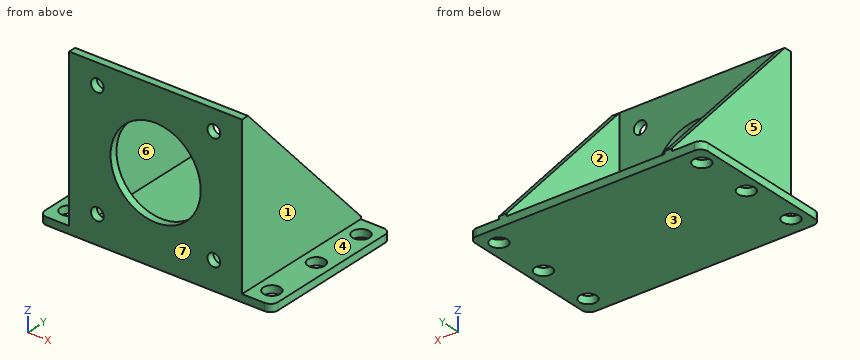
from build123d import *

# Parameters (mm, degrees)
F0_R     = 2.25
F1_DEPTH = 2
F2_W     = 46
F2_H     = 44
F2_R     = 1.7
F2_R_2   = 12
F3_DEPTH = 2
F5_DEPTH = 2
F6_START = -44
F6_DEPTH = 2


with BuildPart() as f1:
    # F0 (on Top) → F1 (new body)
    with BuildSketch(Plane.XY):
        with BuildLine():
            ThreePointArc((0, 2), (0.5857864376, 0.5857864376), (2, 0))
            Line((2, 0), (60, 0))
            ThreePointArc((60, 0), (61.4142135624, 0.5857864376), (62, 2))
            Line((62, 2), (62, 38))
            ThreePointArc((62, 38), (61.4142135624, 39.4142135624), (60, 40))
            Line((60, 40), (2, 40))
            ThreePointArc((2, 40), (0.5857864376, 39.4142135624), (0, 38))
            Line((0, 38), (0, 2))
        make_face()
        with Locations((4, 5)):
            Circle(F0_R, mode=Mode.SUBTRACT)
        with Locations((58, 5)):
            Circle(F0_R, mode=Mode.SUBTRACT)
        with Locations((4, 20)):
            Circle(F0_R, mode=Mode.SUBTRACT)
        with Locations((4, 35)):
            Circle(F0_R, mode=Mode.SUBTRACT)
        with Locations((58, 20)):
            Circle(F0_R, mode=Mode.SUBTRACT)
        with Locations((58, 35)):
            Circle(F0_R, mode=Mode.SUBTRACT)
    extrude(amount=F1_DEPTH)

    # F2 (on Front) → F3 (join)
    with BuildSketch(Plane.XZ):
        with Locations((31, 22)):
            Rectangle(F2_W, F2_H)
        with Locations((15.5, 7.5)):
            Circle(F2_R, mode=Mode.SUBTRACT)
        with Locations((46.5, 7.5)):
            Circle(F2_R, mode=Mode.SUBTRACT)
        with Locations((15.5, 38.5)):
            Circle(F2_R, mode=Mode.SUBTRACT)
        with Locations((31, 23)):
            Circle(F2_R_2, mode=Mode.SUBTRACT)
        with Locations((46.5, 38.5)):
            Circle(F2_R, mode=Mode.SUBTRACT)
    extrude(amount=-F3_DEPTH)

    # F4 (on face) → F5 (join)
    with BuildSketch(Plane(origin=(8, 0, 0), x_dir=(0, -1, 0), z_dir=(-1, 0, 0))):
        Polygon((0, 44), (-2, 44), (-40, 2.6966344009), (-40, 0), (0, 0), align=None)
    extrude(amount=-F5_DEPTH)

    # F4 (on face) → F6 (join)
    with BuildSketch(Plane(origin=(8, 0, 0), x_dir=(0, -1, 0), z_dir=(-1, 0, 0)).offset(F6_START)):
        Polygon((0, 44), (-2, 44), (-40, 2.6966344009), (-40, 0), (0, 0), align=None)
    extrude(amount=-F6_DEPTH)


solid = f1.part
Verification items for the finished model (mm, model axes). Face numbers are marked on the shaded views. A direction names the side the tool comes from. Give positions to 0.01 mm unless a question says otherwise; leave off trailing zeros. Write each loop counter-clockwise with the first axis right and the second up, starting at its lowest first coordinate (ties: lowest second). Pieces come first, ordered by that corner, then holes. Notation, with made-up numbers: (38.25, 0.5) -> (95.25, 0.5) arc R32 ccw to (95.25, 29.5) -> close; hole circle Ø8 at (61, -5.5). An arc over 180 degrees is marked (long way). Use CSV: the item, a comma, the result in double quotes.
(1) Set-up check for the marked faces 4, 5, 6 and 7: record each of +Z, -Z, +X, -X, +Y, -Y from which the full face is reachable in a straight line by a thin tool's end or side.
Derived:
face 4,"+Z, +X, +Y, -Y"
face 5,"+Z, -X, +Y, -Y"
face 6,"+Z, +Y"
face 7,"+Z, -Z, +X, -X, -Y"
(2) Go/stop test with flat-tipped pins: pin 1 (4 mm diameter, centred on y = 24, z = 11, fed in from +X); pin 2 (6 mm diameter, centred on x = 47.5, y = 16, fed in from +Z); pin 3 (1 mm diameter, centred on x = 29, z = 38, fed in from +Y). Record where each tip stops, or that it passes through.
Derived:
pin 1,"stops at x = 54"
pin 2,"stops at z = 2"
pin 3,"stops at y = 2"
(3) Sectioned sample at A-A (x = 58). Record the cut outline in (y, z).
Derived:
outline,"(0, 0) -> (2.75, 0) -> (2.75, 2) -> (0, 2) -> close; (7.25, 0) -> (17.75, 0) -> (17.75, 2) -> (7.25, 2) -> close; (22.25, 0) -> (32.75, 0) -> (32.75, 2) -> (22.25, 2) -> close; (37.25, 0) -> (40, 0) -> (40, 2) -> (37.25, 2) -> close"
(4) Release check for a two-part mould opening along X. For the marked faces 1, 2 and 3 record: +X half, -X half, draft (parallel to the pull), parting line (faces both ways), or undercut.
Derived:
face 1,"+X half"
face 2,"undercut"
face 3,"draft"
(5) Sectioned sample at C-C (z = 24). Record the cut outline in (x, y), plus the area to 3 significant figures.
Derived:
outline,"(8, 0) -> (19.04, 0) -> (19.04, 2) -> (10, 2) -> (10, 20.4) -> (8, 20.4) -> close; (42.96, 0) -> (54, 0) -> (54, 20.4) -> (52, 20.4) -> (52, 2) -> (42.96, 2) -> close"
area,"118 mm^2"
(6) Material ranges on L1, parallel to Y at x = 58, z = 0.65; L2, parallel to Z at x = 15.5, y = 1.3; L3, parallel to X at y = 2.5, z = 27, recorded low to high.
Derived:
L1,"y = 0 to 2.75, 7.25 to 17.75, 22.25 to 32.75, 37.25 to 40"
L2,"z = 0 to 5.8, 9.2 to 36.8, 40.2 to 44"
L3,"x = 8 to 10, 52 to 54"
(7) Sectioned sample at D-D (x = 31). Record the cut outline in (y, z), plus the area to 3 significant figures.
Derived:
outline,"(0, 0) -> (40, 0) -> (40, 2) -> (2, 2) -> (2, 11) -> (0, 11) -> close; (0, 35) -> (2, 35) -> (2, 44) -> (0, 44) -> close"
area,"116 mm^2"
(8) Sectioned sample at B-B (y = 36). Record the cut outline in (x, z), plus the area to 3 significant figures.
Derived:
outline,"(0, 0) -> (1.98, 0) -> (1.98, 2) -> (0, 2) -> close; (6.02, 0) -> (55.98, 0) -> (55.98, 2) -> (54, 2) -> (54, 7.04) -> (52, 7.04) -> (52, 2) -> (10, 2) -> (10, 7.04) -> (8, 7.04) -> (8, 2) -> (6.02, 2) -> close; (60.02, 0) -> (62, 0) -> (62, 2) -> (60.02, 2) -> close"
area,"128 mm^2"
